Geometry: final body of the model. Coordinates: model frame, mm. Give positions to 0.01 mm unless a question says otherwise; leave off trailing zeros. Write each loop counter-clockwise with the first axis right and the second up, starting at its lowest first coordinate (ties: lowest second). Pieces come first, ordered by that corner, then holes.
Q1. Line query: L1, parallel to Y at x = 176, z = 31.5; L2, parallel to Y at x = 58.5, z = 24; L3, parallel to X at y = 72.5, z = 37. Output: solid intervals per line, ascending.
Q2. Cut plane C-C on z = 18.5. Return the cut outline in (x, y).
Q3. Cut plane B-B on y = 92. Return the cut outline in (x, z), plus the area to 3 significant figures.
Q4. Pin query (flat end, axial travel): pin 1 (3 mm diameter, centred on x = 33.5, y = 28, fed in from +Z); pin 2 (1 mm diameter, centred on x = 142.5, z = 53.5, fed in from +Y); pin 3 (1.5 mm diameter, centred on x = 154.5, z = 27, fed in from -Y). Return the tip coordinate at first contact, or that it passes through.
Q5. Cut plane A-A on x = 191. Return the cut outline in (y, z), plus the area to 3 significant figures.
```python
from build123d import *

# Parameters (mm, degrees)
F1_DEPTH = 76.2
F2_R     = 31.75


# Not quite as in the source:
# - a feature names something its author has since deleted; it is built from what else it names


with BuildPart() as f1:
    # F0 (on Top) → F1 (new body)
    with BuildSketch(Plane.XY):
        Polygon((-42.0840979371, 101.6), (0, 0), (246.0318041258, 0), (246.0318041258, 101.6), align=None)
    extrude(amount=F1_DEPTH)

    # F2
    f2_edges = [f1.edges().sort_by_distance(p)[0] for p in [
        (123.015902, 0, 76.2),
        (123.015902, 0, 0),
        (101.973853, 101.6, 76.2),
        (101.973853, 101.6, 0),
    ]]
    fillet(f2_edges, radius=F2_R)


solid = f1.part
```
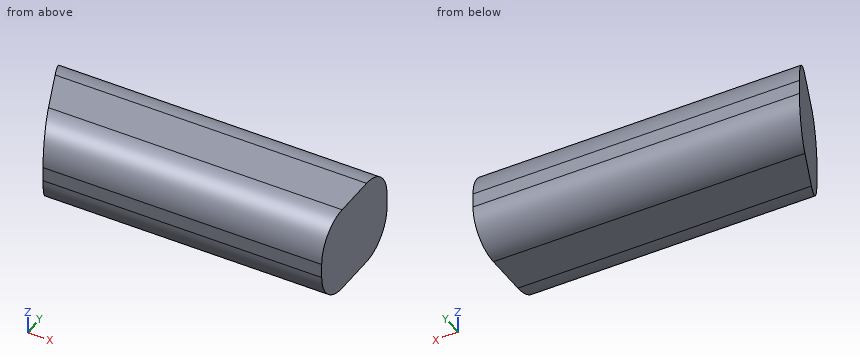
Data:
1. L1: y = 0 to 101.6
1. L2: y = 0.96 to 100.64
1. L3: x = -30.03 to 246.03
2. outline: (-40.88, 98.7) - (-1.2, 2.9) - (246.03, 2.9) - (246.03, 98.7) - close
3. outline: (-38.11, 9) - (246.03, 9) - (246.03, 67.2) - (-38.11, 67.2) - close
3. area: 16,500 mm2
4. pin 1: stops at z = 76.12
4. pin 2: stops at y = 100.43
4. pin 3: stops at y = 0.25
5. outline: (0, 31.75) arc R31.75 ccw to (31.75, 0) - (69.85, 0) arc R31.75 ccw to (101.6, 31.75) - (101.6, 44.45) arc R31.75 ccw to (69.85, 76.2) - (31.75, 76.2) arc R31.75 ccw to (0, 44.45) - close
5. area: 6,880 mm2
